Design review of the part built by this model. Coordinates are the model's own, in mm. Face numbers are marked on the shaded views. Coordinates: 2 decimals unless noted, no trailing zeros. Loops run counter-clockwise (first coordinate to the right, second up) from the corner with the lowest first, then second, coordinate; pieces in that order, holes last. Notation, with made-up numbers: M 5,23 L 64,23 A22 ccw 64,51 Z; hole C 53,12.25 d7. An arc over 180 degrees is marked long. Put each result on its own line as item: value. Start each with the question number.
(1) Take a section at A-A, the plane y = 15.25. Give the boundary of the cut face in (x, z).
(2) Take a section at B-B, the plane z = 0. Give the boundary of the cut face in (x, y).
(3) Take a section at C-C, the plane x = 0. Give the boundary of the cut face in (y, z).
(4) The part is to be moulded in two halves that separate along Z. For the marked faces 1, 2 and 3, say which applies: +Z half, -Z half, draft (parallel to the pull), parting line (faces both ways), or undercut.
(5) Clearance check with a flat-ended pin moving along its axis: pin 1 (1.8 mm diameter, centred on x = 15.505, z = 15.505, fed in from +Y). State where the tip first meets the part, or that it passes through.
(6) Take a section at D-D, the plane y = 24. Give the boundary of the cut face in (x, z) (3 decimals).
(7) For probe 1 along X at (y, z) = (24.5, -4); probe 2 along X at (y, z) = (1.25, -1.5); probe 3 along Z at (x, y) = (8.5, 24.5), list the stretches that pass through material, from the lowest coordinate up. Write a range as [from, to].
```python
from build123d import *

# Parameters (mm, degrees)
SKETCH1_R           = 1.5
SKETCH1_R_2         = 11
BOSS_EXTRUDE1_DEPTH = 26
SKETCH1_3_R         = 1.5
BOSS_EXTRUDE2_DEPTH = 22.5


with BuildPart() as part:
    # Sketch1 → Boss-Extrude1 (new body)
    with BuildSketch(Plane(origin=(0, 0, 0), x_dir=(1, 0, 0), z_dir=(0, 1, 0))):
        Polygon((-15.493145751, 21.15), (-21.15, 15.493145751), (-21.15, -15.493145751), (-15.493145751, -21.15), (15.493145751, -21.15), (21.15, -15.493145751), (21.15, 15.493145751), (15.493145751, 21.15), align=None)
        with Locations(Location((-15.505, -15.505, 0), (0, 0, 90))):
            Circle(SKETCH1_R, mode=Mode.SUBTRACT)
        with Locations(Location((15.505, -15.505, 0), (0, 0, 90))):
            Circle(SKETCH1_R, mode=Mode.SUBTRACT)
        with Locations(Location((0, 0, 0), (0, 0, 90))):
            Circle(SKETCH1_R_2, mode=Mode.SUBTRACT)
        with Locations(Location((-15.505, 15.505, 0), (0, 0, 90))):
            Circle(SKETCH1_R, mode=Mode.SUBTRACT)
        with Locations(Location((15.505, 15.505, 0), (0, 0, 90))):
            Circle(SKETCH1_R, mode=Mode.SUBTRACT)
    extrude(amount=BOSS_EXTRUDE1_DEPTH)

    # Sketch1<3> → Boss-Extrude2 (add)
    with BuildSketch(Plane(origin=(0, 0, 0), x_dir=(1, 0, 0), z_dir=(0, 1, 0))):
        with Locations(Location((15.505, -15.505, 0), (0, 0, 90))):
            Circle(SKETCH1_3_R)
        with Locations(Location((-15.505, -15.505, 0), (0, 0, 90))):
            Circle(SKETCH1_3_R)
        with Locations(Location((15.505, 15.505, 0), (0, 0, 90))):
            Circle(SKETCH1_3_R)
        with Locations(Location((-15.505, 15.505, 0), (0, 0, 90))):
            Circle(SKETCH1_3_R)
    extrude(amount=BOSS_EXTRUDE2_DEPTH)


solid = part.part
```
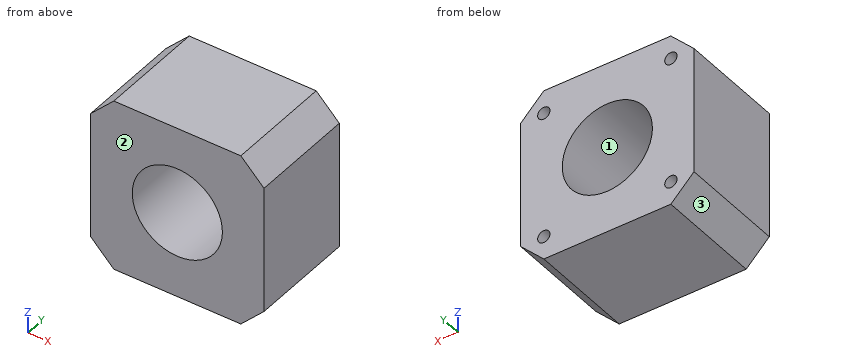
Computed values:
1. outline: M -21.15,-15.49 L -15.49,-21.15 L 15.49,-21.15 L 21.15,-15.49 L 21.15,15.49 L 15.49,21.15 L -15.49,21.15 L -21.15,15.49 Z; hole C 0,0 d22
2. outline: M -21.15,0 L -11,0 L -11,26 L -21.15,26 Z; M 11,0 L 21.15,0 L 21.15,26 L 11,26 Z
3. outline: M 0,-21.15 L 26,-21.15 L 26,-11 L 0,-11 Z; M 0,11 L 26,11 L 26,21.15 L 0,21.15 Z
4. face 1: undercut
4. face 2: draft
4. face 3: -Z half
5. pin 1: stops at y = 22.5
6. outline: M -21.15,-15.493 L -15.493,-21.15 L 15.493,-21.15 L 21.15,-15.493 L 21.15,15.493 L 15.493,21.15 L -15.493,21.15 L -21.15,15.493 Z; hole C -15.505,-15.505 d3; hole C -15.505,15.505 d3; hole C 0,0 d22; hole C 15.505,-15.505 d3; hole C 15.505,15.505 d3
7. probe 1: x = [-21.15, -10.25], [10.25, 21.15]
7. probe 2: x = [-21.15, -10.9], [10.9, 21.15]
7. probe 3: z = [-21.15, -6.98], [6.98, 21.15]
